from build123d import *

# Parameters (mm, degrees)
SKETCH_1_R          = 20.6
EXTRUDE_1_DEPTH     = 4
SKETCH_2_R          = 20.6
EXTRUDE_2_DEPTH     = 1
EXTRUDE_2_TAPER     = 55
SKETCH_3_R          = 19.171851993
EXTRUDE_3_DEPTH     = 3.65
SKETCH_4_R          = 20.6
EXTRUDE_4_DEPTH     = 13.35
EXTRUDE_4_TAPER     = 43.3
SKETCH_5_R          = 5
SKETCH_5_R_2        = 3
EXTRUDE_5_DEPTH     = 4.5
EXTRUDE_START       = 2
EXTRUDE_6_DEPTH     = 2
SKETCH_7_R          = 5.25
EXTRUDE_8_DEPTH     = 4
EXTRUDE_8_TAPER     = 1
SKETCH_8_R          = 2.7
CUT_EXTRUDE_1_DEPTH = 4
SKETCH_9_R          = 1.6
CUT_EXTRUDE_2_DEPTH = 4
SKETCH_10_W         = 3
SKETCH_10_H         = 10
EXTRUDE_9_DEPTH     = 0.1
FILLET_1_R          = 1.5


with BuildPart() as part:
    # 草图1 → 凸台-拉伸1 (new body)
    with BuildSketch(Plane.XY):
        Circle(SKETCH_1_R)
    extrude(amount=EXTRUDE_1_DEPTH)

    # 草图2 → 凸台-拉伸2 (add)
    with BuildSketch(Plane.XY.offset(4)):
        Circle(SKETCH_2_R)
    extrude(amount=EXTRUDE_2_DEPTH, taper=EXTRUDE_2_TAPER)

    # 草图3 → 凸台-拉伸3 (add)
    with BuildSketch(Plane.XY.offset(5)):
        Circle(SKETCH_3_R)
    extrude(amount=EXTRUDE_3_DEPTH)

    # 草图4 → 凸台-拉伸4 (add)
    with BuildSketch(Plane(origin=(0, 0, 0), x_dir=(-1, 0, 0), z_dir=(0, 0, -1))):
        Circle(SKETCH_4_R)
    extrude(amount=EXTRUDE_4_DEPTH, taper=EXTRUDE_4_TAPER)

    # 草图5 → 凸台-拉伸5 (add)
    with BuildSketch(Plane(origin=(0, 0, -13.35), x_dir=(-1, 0, 0), z_dir=(0, 0, -1))):
        Circle(SKETCH_5_R)
        Circle(SKETCH_5_R_2, mode=Mode.SUBTRACT)
    extrude(amount=EXTRUDE_5_DEPTH)

    # 草图6 → 凸台-拉伸6 (add)
    with BuildSketch(Plane.XY.offset(EXTRUDE_START)):
        with BuildLine():
            Line((25, 5.25), (19.069776605, 5.25))
            Line((19.069776605, 5.25), (19.069776605, -5.25))
            Line((19.069776605, -5.25), (25, -5.25))
            ThreePointArc((25, -5.25), (30.25, 0), (25, 5.25))
        make_face()
    extrude_6 = extrude(amount=EXTRUDE_6_DEPTH)

    # 草图7 → 凸台-拉伸8 (add)
    with BuildSketch(Plane(origin=(0, 0, 2), x_dir=(-1, 0, 0), z_dir=(0, 0, -1))):
        with Locations((-25, 0)):
            Circle(SKETCH_7_R)
    extrude_8 = extrude(amount=EXTRUDE_8_DEPTH, taper=EXTRUDE_8_TAPER)

    # 草图8 → 切除-拉伸1 (cut)
    with BuildSketch(Plane.XY.offset(4)):
        with Locations((25, 0)):
            Circle(SKETCH_8_R)
    cut_extrude_1 = extrude(amount=-CUT_EXTRUDE_1_DEPTH, mode=Mode.SUBTRACT)

    # 草图9 → 切除-拉伸2 (cut)
    with BuildSketch(Plane.XY):
        with Locations((25, 0)):
            Circle(SKETCH_9_R)
    cut_extrude_2 = extrude(amount=-CUT_EXTRUDE_2_DEPTH, mode=Mode.SUBTRACT)

    # 镜向1: 凸台-拉伸6, 凸台-拉伸8, 切除-拉伸1, 切除-拉伸2 across plane
    add(extrude_6.mirror(Plane(origin=(0, 0, 0), x_dir=(0, 0, 1), z_dir=(1, 0, 0))))
    add(extrude_8.mirror(Plane(origin=(0, 0, 0), x_dir=(0, 0, 1), z_dir=(1, 0, 0))))
    add(cut_extrude_1.mirror(Plane(origin=(0, 0, 0), x_dir=(0, 0, 1), z_dir=(1, 0, 0))), mode=Mode.SUBTRACT)
    add(cut_extrude_2.mirror(Plane(origin=(0, 0, 0), x_dir=(0, 0, 1), z_dir=(1, 0, 0))), mode=Mode.SUBTRACT)

    # 草图10 → 凸台-拉伸9 (add)
    with BuildSketch(Plane.XY.offset(8.65)):
        with BuildLine():
            Line((-3, 5.196152423), (-4.5, 7.794228634))
            ThreePointArc((-4.5, 7.794228634), (0, -9), (4.5, 7.794228634))
            Line((4.5, 7.794228634), (3, 5.196152423))
            ThreePointArc((3, 5.196152423), (0, -6), (-3, 5.196152423))
        make_face()
        with Locations((0, 6)):
            Rectangle(SKETCH_10_W, SKETCH_10_H)
    extrude(amount=EXTRUDE_9_DEPTH)

    # 圆角1
    fillet_1_edges = [part.edges().sort_by_distance(p)[0] for p in [
        (-3, 5.196152423, 8.7),
        (-4.5, 7.794228634, 8.7),
        (1.5, 1, 8.7),
        (-1.5, 1, 8.7),
        (1.5, 11, 8.7),
        (-1.5, 11, 8.7),
        (4.5, 7.794228634, 8.7),
        (3, 5.196152423, 8.7),
    ]]
    fillet(fillet_1_edges, radius=FILLET_1_R - 0.0001)  # a hair under: the kernel refuses the full size


solid = part.part
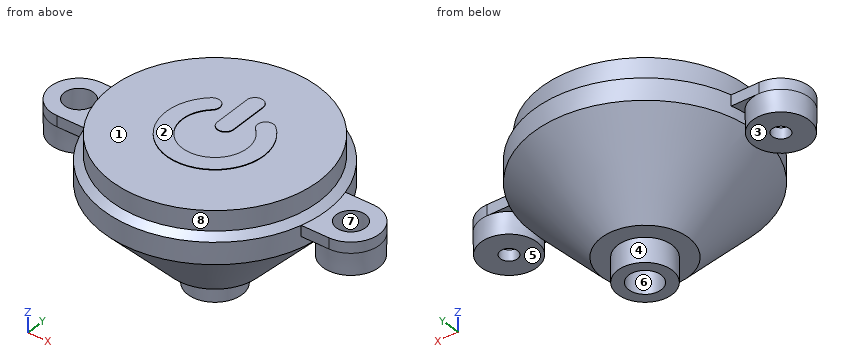
Read the model definition and answer for the solid it produces. Units are mm, in the model's axes. Face numbers are marked on the shaded views. A direction names the side the tool comes from. Round coordinates to 2 decimals unless told otherwise and drop trailing zeros. Order: outer loops, then holes, each group sorted by start corner. A loop starts at its lowest first (then second) coordinate and runs counter-clockwise, first axis right, second up. Notation, with made-up numbers: (55, -24.75) - (74, -24.75) arc R20 cw to (74, 4.25) - close; hole circle Ø11 at (67.25, 75.5). An arc over 180 degrees is marked (long way). Use one line per item in the form item = value. Start each with the question number.
(1) The part is cut by section B-B (z = -10.75). Give the vertices of the cut face in (x, y).
(2) Find the intervals of material crossed by line 1 along Y through (x, z) = (25, -1.25); line 2 along Y through (x, z) = (25, 1.4); line 3 along Y through (x, z) = (7.5, 4), in increasing order. Write a range as from..to.
(3) Flat-ended cylindrical pins translate along their axes: pin 1 Ø0.8 at (x, y) = (-23, -4) entering from -Z; pin 2 Ø4 at (x, z) = (2.5, 2.5) entering from -Y; pin 3 Ø1.6 at (x, z) = (-22, 3.5) entering from -Y. Find the tip coordinate at first contact, or state that the pin passes through.
(4) Determine the mould class of the marked faces 5, 6, 7 and 8 for opening direction Y: +Y half, -Y half, draft (parallel to the pull), parting line (faces both ways), or undercut.
(5) For the marked faces 1, 2, 3 and 4, determine the directions among +Z, -Z, +X, -X, +Y, -Y from which every point of the face is accessible in a straight line to the end or side of a thin tool.
(6) The part is cut by section C-C (z = -6.5). Give the vertices of the cut face in (x, y), then the cut area to 3 significant figures.
(7) The part is cut by section A-A (y = 0). Count the separate pieces of the cut face and the enclosed holes in it, then the cut area to 3 significant figures.
Checked values:
q1.outline = circle Ø20.94 at (0, 0)
q2.line_1 = -5.19..-1.6, 1.6..5.19
q2.line_2 = -5.24..-2.7, 2.7..5.24
q2.line_3 = -19.19..19.19
q3.pin_1 = -2
q3.pin_2 = -20.59
q3.pin_3 = -5.25
q4.face_5 = draft
q4.face_6 = undercut
q4.face_7 = undercut
q4.face_8 = parting line
q5.face_1 = +Z
q5.face_2 = +Z, +X, -X, +Y, -Y
q5.face_3 = -Z, -X, +Y, -Y
q5.face_4 = -Z
q6.outline = circle Ø28.95 at (0, 0)
q6.area = 658 mm^2
q7.separate_pieces = 3
q7.enclosed_holes = 0
q7.area = 807 mm^2
